```python
from build123d import *

# Parameters (mm, degrees)
SKETCH2_W        = 120
SKETCH2_H        = 60
BASE_DEPTH       = 10
SKETCH5_W        = 10
SKETCH5_H        = 60
UPRIGHT_DEPTH    = 70
SKETCH6_R        = 8
SHAFT_HOLE_DEPTH = 50


with BuildPart() as part:
    # Sketch2 → Base (new body)
    with BuildSketch(Plane(origin=(0, 0, 0), x_dir=(1, 0, 0), z_dir=(0, 1, 0))):
        Rectangle(SKETCH2_W, SKETCH2_H)
    extrude(amount=BASE_DEPTH)

    # Sketch5 → Upright (add)
    with BuildSketch(Plane(origin=(0, 10, 0), x_dir=(1, 0, 0), z_dir=(0, 1, 0))):
        with Locations((55, 0)):
            Rectangle(SKETCH5_W, SKETCH5_H)
    extrude(amount=UPRIGHT_DEPTH)

    # Sketch6 → Shaft Hole (cut)
    with BuildSketch(Plane(origin=(60, 0, 0), x_dir=(0, 0, -1), z_dir=(1, 0, 0))):
        with Locations((0, 40)):
            Circle(SKETCH6_R)
    extrude(amount=-SHAFT_HOLE_DEPTH, mode=Mode.SUBTRACT)

    # Mirror 2: part across plane


with BuildPart() as part_1:
    add(part.part)
    add(part.part.mirror(Plane(origin=(0, 0, 0), x_dir=(0, 0, 1), z_dir=(1, 0, 0))))


solid = part_1.part
```
Input: part model. Units: mm. Frame: model coordinates. A direction names the side the tool comes from. Coordinates: 2 decimals unless noted, no trailing zeros. Loops run counter-clockwise (first coordinate to the right, second up) from the corner with the lowest first, then second, coordinate; pieces in that order, holes last. Notation, with made-up numbers: (-3, 88.5) - (23, 88.5) arc R27 ccw to (23, 122.5) - close; hole circle Ø1 at (17.5, 8.5). An arc over 180 degrees is marked (long way). Answer in a Markdown table with one row per item.
(1) Pin query (flat end, axial travel): P1, Ø5, axis at x = -7, z = -14, coming from the +Y side; P2, Ø5, axis at x = 10.5, z = -23, coming from the -Y side. Return the tip coordinate at first contact, or that it passes through.
Model answer:
| item | result |
|---|---|
| P1 | stops at y = 10 |
| P2 | stops at y = 0 |
(2) Material intervals for L1, parallel to X at y = 47.5, z = -6; L2, parallel to Y at x = 53, z = 0; L3, parallel to Y at x = -7, z = 19, sorted ascending. Write a range as from..to.
Model answer:
| item | result |
|---|---|
| L1 | x = -60..-50, 50..60 |
| L2 | y = 0..32, 48..80 |
| L3 | y = 0..10 |
(3) Mould query, pull axis X, two halves, no side actions, for faces 3 (the face through (-60, 31, 0)), 4 (the face through (-55.07, 47.932, 1.041)), 5 (the face through (50, 45, 7)). Classes: pulls with the +X half, pulls with the -X half, needs draft (parallel to the pull), parting line crosses it, or undercut.
Model answer:
| item | result |
|---|---|
| face 3 | pulls with the -X half |
| face 4 | needs draft |
| face 5 | undercut |
(4) Set-up query: faces 1 (the face through (60, 31, 0)), 2 (the face through (-1, 10, 0)). Return all of +Z, -Z, +X, -X, +Y, -Y with unobstructed straight access to the full face (end or side cutting, diameter ignored); none if empty.
Model answer:
| item | result |
|---|---|
| face 1 | +Z, -Z, +X, +Y, -Y |
| face 2 | +Z, -Z, +Y |
(5) Cut plane A-A on y = 56. Output: boundary loops of the cut face in (x, z).
Model answer:
| item | result |
|---|---|
| outline | (-60, -30) - (-50, -30) - (-50, 30) - (-60, 30) - close; (50, -30) - (60, -30) - (60, 30) - (50, 30) - close |
(6) Cut plane D-D on z = -13. Output: boundary loops of the cut face in (x, y), plus the area to 3 significant figures.
Model answer:
| item | result |
|---|---|
| outline | (-60, 0) - (60, 0) - (60, 80) - (50, 80) - (50, 10) - (-50, 10) - (-50, 80) - (-60, 80) - close |
| area | 2,600 mm² |
(7) Cut plane C-C on y = 40. Output: boundary loops of the cut face in (x, z), plus the area to 3 significant figures.
Model answer:
| item | result |
|---|---|
| outline | (-60, -30) - (-50, -30) - (-50, -8) - (-60, -8) - close; (-60, 8) - (-50, 8) - (-50, 30) - (-60, 30) - close; (50, -30) - (60, -30) - (60, -8) - (50, -8) - close; (50, 8) - (60, 8) - (60, 30) - (50, 30) - close |
| area | 880 mm² |
(8) Cut plane B-B on z = 0. Output: boundary loops of the cut face in (x, y), plus the area to 3 significant figures.
Model answer:
| item | result |
|---|---|
| outline | (-60, 0) - (60, 0) - (60, 32) - (50, 32) - (50, 10) - (-50, 10) - (-50, 32) - (-60, 32) - close; (-60, 48) - (-50, 48) - (-50, 80) - (-60, 80) - close; (50, 48) - (60, 48) - (60, 80) - (50, 80) - close |
| area | 2,280 mm² |
